from build123d import *

# Parameters (mm, degrees)
F1_DEPTH = 25.4
F3_D     = 6.35
F5_D     = 6.35
F5_DEPTH = 6.35
F5_TIP   = 1.9077324654
F7_D     = 6.35
F7_DEPTH = 12.7
F7_TIP   = 1.9077324654
F8_R     = 2.54
F9_SIZE  = 2.54


with BuildPart() as f1:
    # F0 (on Top) → F1 (new body)
    with BuildSketch(Plane.XY):
        Polygon((-12.6398103312, -26.1644069105), (0, -26.1644069105), (12.6398103312, -26.1644069105), (12.6398103312, 0), (12.6398103312, 26.1644069105), (0, 26.1644069105), (-12.6398103312, 26.1644069105), (-12.6398103312, 0), align=None)
    extrude(amount=F1_DEPTH)

    # F3 (through all)
    with Locations(Plane.YZ.offset(12.6398103312)):
        with Locations((-13.0822034553, 6.35), (13.0822034553, 6.35)):
            Hole(F3_D / 2)

    # F5
    with Locations(Plane.XZ.offset(26.1644069105)):
        with Locations((-6.3199051656, 6.35), (6.3199051656, 6.35), (0, 19.05)):
            Hole(F5_D / 2, depth=F5_DEPTH)
            with Locations((0, 0, -(F5_DEPTH + F5_TIP / 2))):  # 118° drill point
                Cone(0, F5_D / 2, F5_TIP, mode=Mode.SUBTRACT)

    # F7
    with Locations(Plane.XY.offset(25.4)):
        with Locations((0, 19.6233051829), (0, 6.5411017276), (-6.3199051656, 13.0822034553), (6.3199051656, 13.0822034553), (0, -13.0822034553)):
            Hole(F7_D / 2, depth=F7_DEPTH)
            with Locations((0, 0, -(F7_DEPTH + F7_TIP / 2))):  # 118° drill point
                Cone(0, F7_D / 2, F7_TIP, mode=Mode.SUBTRACT)

    # F8
    f8_edges = [f1.edges().sort_by_distance(p)[0] for p in [
        (12.63981, 0, 25.4),
        (-12.63981, 0, 25.4),
    ]]
    fillet(f8_edges, radius=F8_R)

    # F9
    f9_edges = [f1.edges().sort_by_distance(p)[0] for p in [
        (-12.63981, 0, 0),
        (12.63981, 0, 0),
    ]]
    chamfer(f9_edges, length=F9_SIZE)


solid = f1.part
Verification items for the finished model (mm, model axes). A direction names the side the tool comes from. Give positions to 0.01 mm unless a question says otherwise; leave off trailing zeros. Write each loop counter-clockwise with the first axis right and the second up, starting at its lowest first coordinate (ties: lowest second). Pieces come first, ordered by that corner, then holes. Notation, with made-up numbers: (-21.5, 39) - (-6.5, 39) arc R36 ccw to (-6.5, 78) - close; hole circle Ø4 at (-25, 38.5). An arc over 180 degrees is marked (long way). Answer as CSV lines item,"result". Start each with the question number.
1. Sectioned sample at C-C (z = 3.75). Count the separate pieces of the cut face and the enclosed holes in it, then the cut area to 3 significant figures.
2. Sectioned sample at A-A (y = -22.5). Record the boundary of the cut face in (x, z) (3 decimals).
3. Depth check by flat-ended pin: pin 1 (5.5 mm diameter, centred on x = 0, y = 6.54, fed in from +Z); pin 2 (4 mm diameter, centred on x = 0, z = 19.05, fed in from -Y). Enter the tip coordinate at first touch or a pass-through.
4. Set-up check for faces 1 (the face through (0.413, -9.934, 18.961)), 2 (the face through (4.613, -22.945, 9.027)), 3 (the face through (-11.4, 0.4, 1.3)): record each of +Z, -Z, +X, -X, +Y, -Y from which the full face is reachable in a straight line by a thin tool's end or side.
5. Draft check along X on faces 4 (the face through (-6.439, 12.544, 11.124)), 5 (the face through (-0.177, -10.742, 8.496)), 6 (the face through (12.64, 0, 13)), 7 (the face through (5.769, -18.238, 6.374)). Enter one of: pulls with the +X half, pulls with the -X half, needs draft (parallel to the pull), parting line crosses it, or undercut.
6. Sectioned sample at B-B (z = 14). Record the boundary of the cut face in (x, y) (3 decimals).
7. Thickness scan on line 1 (Y direction, x = 0, z = 22.75); line 2 (X direction, y = -23, z = 6.35); line 3 (Z direction, x = 0, y = -22.25) (3 decimals). Record the ranges inside material, lowest first.
Derived:
1,separate pieces,"3"
1,enclosed holes,"0"
1,area,"1,090 mm²"
2,outline,"(-12.64, 2.54) - (-10.1, 0) - (10.1, 0) - (12.64, 2.54) - (12.64, 22.86) arc R2.54 ccw to (10.1, 25.4) - (-10.1, 25.4) arc R2.54 ccw to (-12.64, 22.86) - close; hole circle Ø6.35 at (-6.32, 6.35); hole circle Ø6.35 at (0, 19.05); hole circle Ø6.35 at (6.32, 6.35)"
3,pin 1,"z = 12.45"
3,pin 2,"y = -19.11"
4,face 1,"+Z"
4,face 2,"-Y"
4,face 3,"-Z, -X, +Y, -Y"
5,face 4,"undercut"
5,face 5,"needs draft"
5,face 6,"pulls with the +X half"
5,face 7,"undercut"
6,outline,"(-12.64, -26.164) - (12.64, -26.164) - (12.64, 26.164) - (-12.64, 26.164) - close; hole circle Ø6.35 at (-6.32, 13.082); hole circle Ø6.35 at (0, -13.082); hole circle Ø6.35 at (0, 6.541); hole circle Ø6.35 at (0, 19.623); hole circle Ø6.35 at (6.32, 13.082)"
7,line 1,"-26.16 to -16.26, -9.91 to 3.37, 9.72 to 16.45, 22.8 to 26.16"
7,line 2,"-12.64 to -9.49, -3.14 to 3.14, 9.49 to 12.64"
7,line 3,"0 to 15.875, 22.225 to 25.4"
